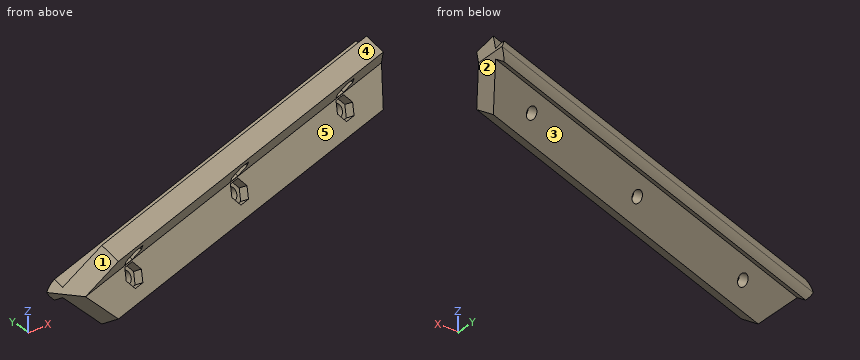
```python
from build123d import *

# Parameters (mm, degrees)
BOSS_EXTRUDE1_DEPTH = 76.2
CUT_EXTRUDE2_START  = -64.90373811
CUT_EXTRUDE2_DEPTH  = 68.722745412
SKETCH4_R           = 1.7145
CUT_EXTRUDE3_DEPTH  = 2.5
SKETCH6_R           = 1.7145
CUT_EXTRUDE4_DEPTH  = 50.868554483


with BuildPart() as part:
    # Sketch2 → Boss-Extrude1 (new body, symmetric)
    with BuildSketch(Plane(origin=(-61.535605536, -23.504509797, 0), x_dir=(0, 0, 1), z_dir=(-0.934172359, -0.35682209, 0))):
        with BuildLine():
            Line((-1.374815328, -3.984929137), (-2.776940204, -1.716243431))
            ThreePointArc((-2.776940204, -1.716243431), (-1.443408604, -1.128416568), (0, -0.927372913))
            Line((0, -0.927372913), (0, -9.404564037))
            Line((0, -9.404564037), (-7.662421822, -14.140201159))
            Line((-7.662421822, -14.140201159), (-10.466145843, -9.603680398))
            Line((-10.466145843, -9.603680398), (-1.374815328, -3.984929137))
        make_face()
    boss_extrude1 = extrude(amount=BOSS_EXTRUDE1_DEPTH, both=True)

    # Mirror4: Boss-Extrude1 across plane
    add(boss_extrude1.mirror(Plane(origin=(13.00408441, -5.100150327, 0), x_dir=(1, 0, 0), z_dir=(0, 0, 1))))

    # Sketch3 → Cut-Extrude2 (cut)
    with BuildSketch(Plane(origin=(0, 0, 0), x_dir=(1, 0, 0), z_dir=(0, 1, 0)).offset(CUT_EXTRUDE2_START)):
        Polygon((-6.04263212, 10.466145843), (0, 0), (-6.04263212, -10.466145843), (57.45736788, -10.466145843), (57.45736788, 10.466145843), align=None)
    cut_extrude2 = extrude(amount=CUT_EXTRUDE2_DEPTH, mode=Mode.SUBTRACT)

    # Mirror5: Cut-Extrude2 across plane
    add(cut_extrude2.mirror(Plane(origin=(-61.535605536, -23.504509797, 0), x_dir=(0, 0, 1), z_dir=(0.934172359, 0.35682209, 0))), mode=Mode.SUBTRACT)

    # Sketch4 → Cut-Extrude3 (cut)
    with BuildSketch(Plane(origin=(2.428247993, -6.357235778, 4.205848897), x_dir=(0.952821564, 0.253145264, -0.167476992), z_dir=(0.303530999, -0.794654472, 0.525731112))):
        Polygon((-109.695418088, -30.215326769), (-107.597357756, -32.598911501), (-104.48408266, -31.973730321), (-103.468867896, -28.964964409), (-105.566928228, -26.581379677), (-108.680203324, -27.206560857), align=None)
        with Locations((-106.582142992, -29.590145589)):
            Circle(SKETCH4_R, mode=Mode.SUBTRACT)
        Polygon((-66.115420605, -21.46396577), (-64.017360273, -23.847550502), (-60.904085176, -23.222369322), (-59.888870412, -20.21360341), (-61.986930744, -17.830018678), (-65.100205841, -18.455199858), align=None)
        with Locations((-63.002145509, -20.83878459)):
            Circle(SKETCH4_R, mode=Mode.SUBTRACT)
        Polygon((-22.535423121, -12.712604771), (-20.437362789, -15.096189503), (-17.324087693, -14.471008323), (-16.308872929, -11.462242411), (-18.406933261, -9.078657679), (-21.520208357, -9.703838859), align=None)
        with Locations((-19.422148025, -12.087423591)):
            Circle(SKETCH4_R, mode=Mode.SUBTRACT)
    cut_extrude3 = extrude(amount=-CUT_EXTRUDE3_DEPTH, mode=Mode.SUBTRACT)

    # Sketch6 → Cut-Extrude4 (cut, through all)
    with BuildSketch(Plane(origin=(2.428247993, -6.357235778, 4.205848897), x_dir=(0.952821564, 0.253145264, -0.167476992), z_dir=(0.303530999, -0.794654472, 0.525731112))):
        with Locations((-106.582142992, -29.590145589)):
            Circle(SKETCH6_R)
        with Locations((-63.002145509, -20.83878459)):
            Circle(SKETCH6_R)
        with Locations((-19.422148025, -12.087423591)):
            Circle(SKETCH6_R)
    cut_extrude4 = extrude(amount=-CUT_EXTRUDE4_DEPTH, mode=Mode.SUBTRACT)

    # Mirror6: Cut-Extrude3, Cut-Extrude4 across plane
    add(cut_extrude3.mirror(Plane.XY), mode=Mode.SUBTRACT)
    add(cut_extrude4.mirror(Plane.XY), mode=Mode.SUBTRACT)


solid = part.part
```
Input: part model. Units: mm. Frame: model coordinates. Face numbers are marked on the shaded views. A direction names the side the tool comes from. Coordinates: 2 decimals unless noted, no trailing zeros. Put each result on its own line as item: value. Start each with the question number.
1) Contact query for flat-ended pins moving along their axis: pin 1 (3 mm diameter, centred on x = -36.5, y = -18, fed in from +Z); pin 2 (6 mm diameter, centred on x = -17.5, z = 2.5, fed in from -Y); pin 3 (8 mm diameter, centred on x = -98, y = -36.5, fed in from +Z). Output: stop coordinate, or through.
2) Ray query, L1, parallel to Y at x = -108, z = 6.5; L2, parallel to Z at x = -69.5, y = -37; L3, parallel to Z at x = -103, y = -49.5. Return the intervals inside material, ascending.
3) Mould query, pull axis Y, two halves, no side actions, for the marked faces 1, 2 and 3. Classes: pulls with the +Y half, pulls with the -Y half, needs draft (parallel to the pull), parting line crosses it, or undercut.
4) Reachability of the marked faces 4 and 5 from +Z, -Z, +X, -X, +Y, -Y: full face, straight path, thin tool, end or side. Return the list, or none.
Resolved:
1. pin 1: stops at z = 3.49
1. pin 2: stops at y = -20.7
1. pin 3: stops at z = 2.78
2. L1: y = -55.62 to -48.91
2. L2: z = -10.37 to -0.58, 0.58 to 10.37
2. L3: z = -10.28 to -0.14, 0.14 to 10.28
3. face 1: pulls with the -Y half
3. face 2: needs draft
3. face 3: undercut
4. face 4: +Z, +X, -Y
4. face 5: +X, -Y
